Here's how the part is built. I have some questions about the finished solid (model axes, mm). Face numbers are marked on the shaded views. A direction names the side the tool comes from. Coordinates: 2 decimals unless noted, no trailing zeros. Write each loop counter-clockwise with the first axis right and the second up, starting at its lowest first coordinate (ties: lowest second). Pieces come first, ordered by that corner, then holes. Notation, with made-up numbers: M -2.75,-37 L 20.25,-37 A15 ccw 20.25,-9 Z; hole C 9,41 d7. An arc over 180 degrees is marked long. Use a Markdown table: item, result.
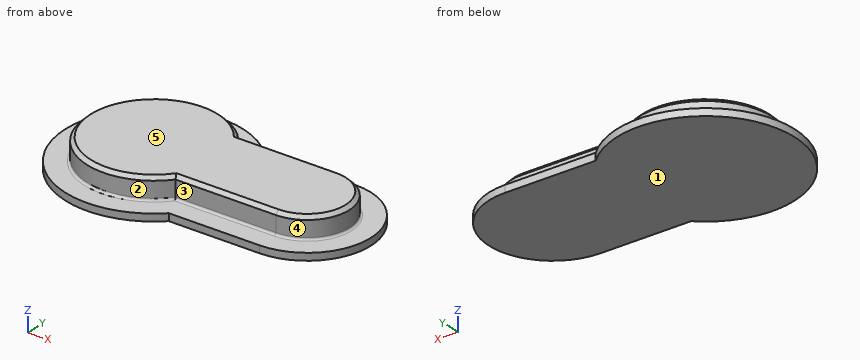
```python
from build123d import *

# Parameters (mm, degrees)
F1_DEPTH = 3
F3_DEPTH = 1
F4_SIZE  = 0.5
F5_R     = 0.3


with BuildPart() as f1:
    # F0 (on Top) → F1 (new body)
    with BuildSketch(Plane.XY):
        with BuildLine():
            Line((21.1, 5.8), (7.2698005475, 5.8))
            ThreePointArc((7.2698005475, 5.8), (-9.3, 0), (7.2698005475, -5.8))
            Line((7.2698005475, -5.8), (21.1, -5.8))
            ThreePointArc((21.1, -5.8), (26.9, 0), (21.1, 5.8))
        make_face()
    extrude(amount=F1_DEPTH)

    # F2 (on face) → F3 (join)
    with BuildSketch(Plane(origin=(0, 0, 0), x_dir=(1, 0, 0), z_dir=(0, 0, -1))):
        with BuildLine():
            ThreePointArc((21.1, -8.8), (29.9, 0), (21.1, 8.8))
            Line((21.1, 8.8), (8.5936022715, 8.8))
            ThreePointArc((8.5936022715, 8.8), (-12.3, 0), (8.5936022715, -8.8))
            Line((8.5936022715, -8.8), (21.1, -8.8))
        make_face()
    extrude(amount=F3_DEPTH)

    # F4
    f4_edges = [f1.edges().sort_by_distance(p)[0] for p in [
        (14.1849, -5.8, 3),
        (26.9, 0, 3),
        (14.1849, 5.8, 3),
        (-9.3, 0, 3),
    ]]
    chamfer(f4_edges, length=F4_SIZE)

    # F5
    f5_edges = [f1.edges().sort_by_distance(p)[0] for p in [
        (-9.3, 0, 0),
        (14.1849, -5.8, 0),
        (26.9, 0, 0),
        (14.1849, 5.8, 0),
    ]]
    fillet(f5_edges, radius=F5_R)


solid = f1.part
```
1. Will these pins go through, and if not, where does the flat tip stop? pin 1 Ø1.5 at (y, z) = (8, 0) entering from -X; pin 2 Ø1.1 at (x, z) = (15, 1.5) entering from +Y; pin 3 Ø0.8 at (x, z) = (17, -0.5) entering from -Y.
Answers follow:
| item | result |
|---|---|
| pin 1 | stops at x = -9.94 |
| pin 2 | stops at y = 5.8 |
| pin 3 | stops at y = -8.8 |
2. I need wall thicknesses on probe 1 along Z at (x, y) = (-5, 9.25); probe 2 along Z at (x, y) = (-5, 7.25); probe 3 along Y at (x, z) = (14, 0.75). Which ranges of each line are inside material? Lowest first, please.
Answers follow:
| item | result |
|---|---|
| probe 1 | z = -1 to 0 |
| probe 2 | z = -1 to 2.99 |
| probe 3 | y = -5.8 to 5.8 |
3. Suppose I cut it at A-A on y = 0. Write out the boundary of the cut face in (x, z).
Answers follow:
| item | result |
|---|---|
| outline | M -12.3,-1 L 29.9,-1 L 29.9,0 L 27.2,0 A0.3 cw 26.9,0.3 L 26.9,2.5 L 26.4,3 L -8.8,3 L -9.3,2.5 L -9.3,0.3 A0.3 cw -9.6,0 L -12.3,0 Z |
4. Which directions (+Z, -Z, +X, -X, +Y, -Y) give clear straight access to the entire face, cutting with the end or side of a thin tool? Please do the marked faces 1, 2, 3, 4 and 5.
Answers follow:
| item | result |
|---|---|
| face 1 | -Z, +X, -X, +Y, -Y |
| face 2 | +Z |
| face 3 | +Z, +X, -Y |
| face 4 | +Z, +X |
| face 5 | +Z, +X, -X, +Y, -Y |
5. Suppose I cut it at B-B on z = 1.15. Write out the boundary of the cut face in (x, y).
Answers follow:
| item | result |
|---|---|
| outline | M 7.27,-5.8 L 21.1,-5.8 A5.8 ccw 21.1,5.8 L 7.27,5.8 A9.3 ccw long Z |
6. Suppose I cut it at C-C on y = 10. Write out the boundary of the cut face in (x, z), and give its area (3 significant figures).
Answers follow:
| item | result |
|---|---|
| outline | M -7.16,-1 L 7.16,-1 L 7.16,0 L -7.16,0 Z |
| area | 14.3 mm2 |
